```python
from build123d import *

# Parameters (mm, degrees)
BOSS_EXTRU_1_DEPTH              = 100
DIAM_TRE_DU_PER_AGE_4_5_4_5_1_D = 4.5
BOSS_EXTRU_2_DEPTH              = 40


with BuildPart() as part:
    # Esquisse1 → Boss.-Extru.1 (new, symmetric)
    with BuildSketch(Plane.XY):
        Polygon((-13.777077185, 10), (-8.777077185, 10), (-8.777077185, 14.5), (0, 14.5), (0, 0), (-13.777077185, 0), align=None)
    extrude(amount=BOSS_EXTRU_1_DEPTH, both=True)

    # Diamètre du perçage Ø4.5 (4.5)1 (through all)
    with Locations(Plane(origin=(0, 14.5, 0), x_dir=(1, 0, 0), z_dir=(0, 1, 0))):
        with Locations((-4.388538592, -74.166666667), (-4.388538592, 84.166666667), (-4.388538592, 52.5), (-4.388538592, 20.833333333), (-4.388538592, -10.833333333), (-4.388538592, -42.5)):
            Hole(DIAM_TRE_DU_PER_AGE_4_5_4_5_1_D / 2)

    # Esquisse4 → Boss.-Extru.2 (add)
    with BuildSketch(Plane.XY.offset(100)):
        Polygon((-13.777077185, 10), (-13.777077185, 0), (0, 0), (0, 14.5), (-8.777077185, 14.5), (-8.777077185, 10), align=None)
    extrude(amount=BOSS_EXTRU_2_DEPTH)


solid = part.part
```
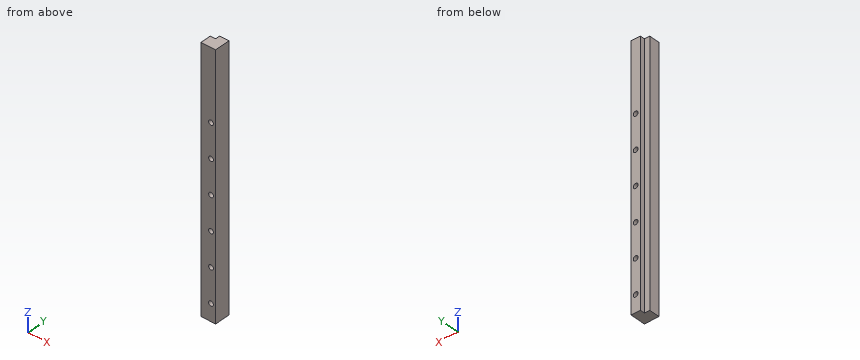
Can you work these out from the model? Positions are in its coordinate system, mm. Round coordinates to 2 decimals unless told otherwise and drop trailing zeros. Order: outer loops, then holes, each group sorted by start corner. A loop starts at its lowest first (then second) coordinate and runs counter-clockwise, first axis right, second up. Notation, with made-up numbers: (78.25, 83) -> (134.25, 83) arc R20 cw to (134.25, 105) -> close; hole circle Ø11 at (81.5, -16). An arc over 180 degrees is marked (long way). Return JSON: item names as keys, results as strings. Group by question number.
1. Will these pins go through, and if not, where does the flat tip stop? pin 1 (5 mm diameter, centred on x = -4.39, z = 74.17, fed in from -Y); pin 2 (2 mm diameter, centred on y = 13, z = 59, fed in from -X).
2. If we section it at D-D, the plane z = -78: Write out the boundary of the cut face in (x, y).
3. If we section it at C-C, the plane x = -11.25: Write out the boundary of the cut face in (y, z), then the cut area to 3 significant figures.
4. I need wall thicknesses on line 1 (Y direction, x = -13, z = 44.5); line 2 (X direction, y = 6.75, z = -21); line 3 (X direction, y = 10.75, z = -10). Which ranges of each line are inside material? Lowest first, please. Write a range as [from, to].
5. If we section it at A-A, the plane z = -52.5: Write out the boundary of the cut face in (x, y), then the cut area to 3 significant figures.
6. If we section it at B-B, the plane y = 5: Write out the boundary of the cut face in (x, z).
Output values:
{
 "1": {"pin 1": "y = 0", "pin 2": "x = -8.78"},
 "2": {"outline": "(-13.78, 0) -> (0, 0) -> (0, 14.5) -> (-8.78, 14.5) -> (-8.78, 10) -> (-13.78, 10) -> close"},
 "3": {"outline": "(0, -100) -> (10, -100) -> (10, 140) -> (0, 140) -> close", "area": "2,400 mm²"},
 "4": {"line 1": "[0, 10]", "line 2": "[-13.78, -6.63], [-2.14, 0]", "line 3": "[-8.78, 0]"},
 "5": {"outline": "(-13.78, 0) -> (-6.64, 0) -> (-6.64, 14.5) -> (-8.78, 14.5) -> (-8.78, 10) -> (-13.78, 10) -> close; (-2.14, 0) -> (0, 0) -> (0, 14.5) -> (-2.14, 14.5) -> close", "area": "112 mm²"},
 "6": {"outline": "(-13.78, -100) -> (0, -100) -> (0, 140) -> (-13.78, 140) -> close; hole circle Ø4.5 at (-4.39, -84.17); hole circle Ø4.5 at (-4.39, -52.5); hole circle Ø4.5 at (-4.39, -20.83); hole circle Ø4.5 at (-4.39, 10.83); hole circle Ø4.5 at (-4.39, 42.5); hole circle Ø4.5 at (-4.39, 74.17)"}
}
